Could you check a few things on this model? Use its own coordinates, in mm. A direction names the side the tool comes from. Give positions to 0.01 mm unless a question says otherwise; leave off trailing zeros. Write each loop counter-clockwise with the first axis right and the second up, starting at its lowest first coordinate (ties: lowest second). Pieces come first, ordered by that corner, then holes. Notation, with made-up numbers: (18, 7.5) - (58, 7.5) arc R20 ccw to (58, 43.5) - close; hole circle Ø6 at (45, 16). An arc over 180 degrees is marked (long way). Answer as CSV lines item,"result". Start each with the question number.
Q1. On a 3-axis mill with a long thin cutter (end or side, diameter ignored), from which of +Z, -Z, +X, -X, +Y, -Y can I reach the whole of each face in a straight line? I mean faces 1 (the face through (-457.2, 0, 0)), 2 (the face through (104.38, -5.69, -604.69)), 3 (the face through (-225.4, 25.039, -7.885)). Say none if no direction works.
Q2. If I drill on line 1 along X through (y, z) = (8, -663.5); line 2 along X through (y, z) = (6.5, -115); line 3 along Z through (x, y) = (-333.5, -2), over which ranges is the centre line in solid material (lowest first)?
Q3. Imagine slicing it at A-A on y = 0. List the corners of the cut face in (x, z) for me.
Q4. Imagine slicing it at C-C on z = -117.5. List the corners of the cut face in (x, y) for me, and give its area (3 significant figures).
Q5. Imagine slicing it at B-B on x = -67.5. List the corners of the cut face in (y, z) for me.
Q6. Will these pins go through, and if not, where does the flat tip stop? pin 1 Ø6 at (y, z) = (-8.5, -881.5) entering from +X; pin 2 Ø10 at (x, y) = (-225.5, -7) entering from +Z; pin 3 Ø1.5 at (x, y) = (-57, -14.5) entering from +Z.
```python
from build123d import *

# Parameters (mm, degrees)
F0_R     = 26.2509
F3_DEPTH = 1066.8
F4_DEPTH = 457.2


with BuildPart() as f2:
    # F2: sweep along a path in F1
    with BuildLine(Plane.XZ) as f2_path:
        ThreePointArc((0, 0), (55.6865682067, -23.0661317933), (78.7527, -78.7527))
    # F0 (on Right) → F2 (sweep)
    with BuildSketch(Plane.YZ):
        Circle(F0_R)
    sweep(path=f2_path.line)

    # F3 (add): a face of the model
    f3_faces = [f2.faces().sort_by_distance(p)[0] for p in [
        (78.7527, 0, -78.7527),
    ]]
    extrude(f3_faces, amount=F3_DEPTH)

    # F4 (add): a face of the model
    f4_faces = [f2.faces().sort_by_distance(p)[0] for p in [
        (0, 0, 0),
    ]]
    extrude(f4_faces, amount=F4_DEPTH)


solid = f2.part
```
Conclusion:
1,face 1,"+Z, -Z, -X, +Y, -Y"
1,face 2,"-Z"
1,face 3,"-X"
2,line 1,"53.75 to 103.75"
2,line 2,"53.32 to 104.19"
2,line 3,"-26.17 to 26.17"
3,outline,"(-457.2, -26.25) - (0, -26.25) arc R52.5 cw to (52.5, -78.75) - (52.5, -1145.55) - (105, -1145.55) - (105, -78.75) arc R105 ccw to (0, 26.25) - (-457.2, 26.25) - close"
4,outline,"circle Ø52.5 at (78.75, 0)"
4,area,"2,160 mm^2"
5,outline,"circle Ø52.5 at (0, 0)"
6,pin 1,"x = 104.42"
6,pin 2,"z = 26.17"
6,pin 3,"z = 22.36"
